from build123d import *

# Parameters (mm, degrees)
SKETCH1_R           = 45
BOSS_EXTRUDE1_DEPTH = 20
SKETCH2_R           = 50
SKETCH2_R_2         = 45
BOSS_EXTRUDE2_DEPTH = 5


with BuildPart() as part:
    # Sketch1 → Boss-Extrude1 (new body)
    with BuildSketch(Plane.XY):
        Circle(SKETCH1_R)
    extrude(amount=BOSS_EXTRUDE1_DEPTH)

    # Sketch2 → Boss-Extrude2 (add)
    # profile 1 of 2: a face of its own
    with BuildSketch(Plane(origin=(0, 0, 0), x_dir=(-1, 0, 0), z_dir=(0, 0, -1))):
        with BuildLine():
            Line((115.311288741, 20), (40.311288741, 20))
            ThreePointArc((40.311288741, 20), (43.812144397, 10.271124735), (45, 0))
            ThreePointArc((45, 0), (43.812144397, -10.271124735), (40.311288741, -20))
            Line((40.311288741, -20), (115.311288741, -20))
            ThreePointArc((115.311288741, -20), (111.137045691, 0), (115.311288741, 20))
        make_face()
    # profile 2 of 2: a face of its own
    with BuildSketch(Plane(origin=(0, 0, 0), x_dir=(-1, 0, 0), z_dir=(0, 0, -1))):
        with Locations((161.137045691, 0)):
            Circle(SKETCH2_R)
        with Locations((161.137045691, 0)):
            Circle(SKETCH2_R_2, mode=Mode.SUBTRACT)
    extrude(amount=-BOSS_EXTRUDE2_DEPTH)


solid = part.part
Could you check a few things on this model? Use its own coordinates, in mm. A direction names the side the tool comes from. Coordinates: 2 decimals unless noted, no trailing zeros. Write each loop counter-clockwise with the first axis right and the second up, starting at its lowest first coordinate (ties: lowest second). Pieces come first, ordered by that corner, then holes. Notation, with made-up numbers: (36, 29) - (54, 29) arc R34 ccw to (54, 68) - close; hole circle Ø10 at (-9, 15.5). An arc over 180 degrees is marked (long way). Write item = value, one per line.
1) Suppose I cut it at B-B on x = -142. Please give me the cut outline in (y, z), plus the area to 3 significant figures.
Result set:
outline = (-46.19, 0) - (-40.73, 0) - (-40.73, 5) - (-46.19, 5) - close; (40.73, 0) - (46.19, 0) - (46.19, 5) - (40.73, 5) - close
area = 54.6 mm2
2) For faces 3 (the flat face through (-77, -20, 2)), 4 (the flat face through (-78, 20, 2)), 5 (the flat face through (-1, 1, 20)), which set-ups out of +Z, -Z, +X, -X, +Y, -Y let a thin tool reach every point of the face, with its end or its side?
Result set:
face_3 = +Z, -Z, -Y
face_4 = +Z, -Z, +Y
face_5 = +Z, +X, -X, +Y, -Y
3) Suppose I cut it at D-D on y = -24. Please give me the cut outline in (x, z).
Result set:
outline = (-205, 0) - (-199.2, 0) - (-199.2, 5) - (-205, 5) - close; (-123.07, 0) - (-117.27, 0) - (-117.27, 5) - (-123.07, 5) - close; (-38.07, 0) - (38.07, 0) - (38.07, 20) - (-38.07, 20) - close
4) Please list where these lines run through material, in increasing order: line 1 (Z direction, x = -106, y = 17.5); line 2 (X direction, y = 13, z = 1.5); line 3 (X direction, y = 22.5, z = 10.25). Write a range as [from, to].
Result set:
line_1 = [0, 5]
line_2 = [-209.42, -204.22], [-118.06, 43.08]
line_3 = [-38.97, 38.97]
5) We'd pull the mould along X, two halves only. Please class faces 1 (the flat face through (-53, 1, 0)), 2 (the cylindrical face through (-202.706, -17.235, 2.465)): +X half, -X half, draft (parallel to the pull), parting line (faces both ways), or undercut.
Result set:
face_1 = draft
face_2 = undercut
6) Will these pins go through, and if not, where does the flat tip stop? pin 1 Ø4 at (y, z) = (35, 17) entering from +X; pin 2 Ø1.5 at (x, z) = (-86.5, 3.5) entering from -Y; pin 3 Ø5.5 at (x, z) = (-86.5, 2.5) entering from +Y; pin 4 Ø10 at (x, z) = (-129.5, 11.5) entering from -Y.
Result set:
pin_1 = 30.59
pin_2 = -20
pin_3 = 20
pin_4 = through
7) Suppose I cut it at C-C on z = 2.25. Please give me the cut outline in (x, y), plus the area to 3 significant figures.
Result set:
outline = (-115.31, -20) - (-40.31, -20) arc R45 ccw (long way) to (-40.31, 20) - (-115.31, 20) arc R50 ccw (long way) to start; hole circle Ø90 at (-161.14, 0)
area = 10,600 mm2
8) Suppose I cut it at A-A on y = 0. Please give me the cut outline in (x, z).
Result set:
outline = (-211.14, 0) - (-206.14, 0) - (-206.14, 5) - (-211.14, 5) - close; (-116.14, 0) - (45, 0) - (45, 20) - (-45, 20) - (-45, 5) - (-116.14, 5) - close
